```python
from build123d import *

# Parameters (mm, degrees)
SKETCH1_W           = 46
SKETCH1_H           = 46
BOSS_EXTRUDE3_DEPTH = 11
SKETCH3_R           = 17.5
SKETCH3_R_2         = 16
BOSS_EXTRUDE5_DEPTH = 3
SKETCH6_R           = 12.5
CUT_EXTRUDE2_DEPTH  = 40.268307832
FILLET1_R           = 3


with BuildPart() as part:
    # Sketch1 → Boss-Extrude3 (new, symmetric)
    with BuildSketch(Plane.XY):
        Rectangle(SKETCH1_W, SKETCH1_H)
    extrude(amount=BOSS_EXTRUDE3_DEPTH, both=True)

    # Sketch3 → Boss-Extrude5 (add)
    with BuildSketch(Plane.XY.offset(11)):
        Circle(SKETCH3_R)
        Circle(SKETCH3_R_2, mode=Mode.SUBTRACT)
    boss_extrude5 = extrude(amount=BOSS_EXTRUDE5_DEPTH)

    # Sketch6 → Cut-Extrude2 (cut, through all)
    with BuildSketch(Plane.XY.offset(11)):
        Circle(SKETCH6_R)
    extrude(amount=-CUT_EXTRUDE2_DEPTH, mode=Mode.SUBTRACT)

    # Mirror1: Boss-Extrude5 across plane
    add(boss_extrude5.mirror(Plane.XY))

    # Fillet1
    fillet1_edges = [part.edges().sort_by_distance(p)[0] for p in [
        (-17.5, 0, 11),
        (-17.5, 0, -11),
    ]]
    fillet(fillet1_edges, radius=FILLET1_R - 0.0001)  # a hair under: the kernel refuses the full size

    # Sketch9 → Revolve1 (revolve)
    with BuildSketch(Plane.XY):
        Polygon((-23, 0), (-23, 8), (-35, 8), (-35, 6), (-45, 6), (-45, 0), align=None)
    revolve1 = revolve(axis=Axis((-23, 0, 0), (-1, 0, 0)))

    # Mirror2: Revolve1 across plane
    add(revolve1.mirror(Plane(origin=(0, 0, 0), x_dir=(0, 0, 1), z_dir=(1, 0, 0))))


solid = part.part
```
Here's how the part is built. I have some questions about the finished solid (model axes, mm). A direction names the side the tool comes from. Give positions to 0.01 mm unless a question says otherwise; leave off trailing zeros. Loops run counter-clockwise (first coordinate to the right, second up) from the corner with the lowest first, then second, coordinate; pieces in that order, holes last. Notation, with made-up numbers: M 17.5,1.5 L 25.5,1.5 A17 ccw 25.5,23.5 Z; hole C 65.25,52 d10. An arc over 180 degrees is marked long. Put each result on its own line as item: value. Start each with the question number.
(1) I need wall thicknesses on line 1 along Y through (x, z) = (0, 6); line 2 along Z through (x, y) = (-17.5, -17.5); line 3 along Z through (x, y) = (-27.5, 0.5). Which ranges of each line are inside material? Lowest first, please. Write a range as [from, to].
(2) I want a section at B-B on z = 2.5. Please give me the cut outline in (x, y), then the cut area to 3 significant figures.
(3) I want a section at C-C on x = 24.5. Please give me the cut outline in (y, z), then the cut area to 3 significant figures.
(4) I want a section at D-D on z = 7. Please give me the cut outline in (x, y).
(5) If we mould it in two halves opening along Y, with no side actions, what happens to faces 4 (the cylindrical face through (-3.47, -15.62, -12.48)), 5 (the cylindrical face through (40, -6, 0)), 6 (the flat face through (-45, 0, 0))? For each: +Y half, -Y half, draft (parallel to the pull), parting line (faces both ways), or undercut.
(6) For faces 1 (the cylindrical face through (29.08, -1.73, 7.81)), 2 (the flat face through (-35, -2, -6)), 3 (the flat face through (-21, 0, -11)), which set-ups out of +Z, -Z, +X, -X, +Y, -Y let a thin tool reach every point of the face, with its end or its side?
(7) Will these pins go through, and if not, where does the flat tip stop? pin 1 Ø1.5 at (y, z) = (-9.5, -10.5) entering from +X; pin 2 Ø4 at (y, z) = (-16, -1.5) entering from -X; pin 3 Ø4 at (x, z) = (-26, -8.5) entering from -Y.
Answer block:
1. line 1: [-23, -12.5], [12.5, 23]
1. line 2: [-11, 11]
1. line 3: [-7.98, 7.98]
2. outline: M -45,-5.45 L -35,-5.45 L -35,-7.6 L -23,-7.6 L -23,-23 L 23,-23 L 23,-7.6 L 35,-7.6 L 35,-5.45 L 45,-5.45 L 45,5.45 L 35,5.45 L 35,7.6 L 23,7.6 L 23,23 L -23,23 L -23,7.6 L -35,7.6 L -35,5.45 L -45,5.45 Z; hole C 0,0 d25
2. area: 2,210 mm^2
3. outline: C 0,0 d16
3. area: 201 mm^2
4. outline: M -35,-3.87 L -23,-3.87 L -23,-23 L 23,-23 L 23,-3.87 L 35,-3.87 L 35,3.87 L 23,3.87 L 23,23 L -23,23 L -23,3.87 L -35,3.87 Z; hole C 0,0 d25
5. face 4: undercut
5. face 5: parting line
5. face 6: draft
6. face 1: +X
6. face 2: -X
6. face 3: -Z
7. pin 1: x = 23
7. pin 2: x = -23
7. pin 3: y = -4.66
